Part print with two shaded views. Sizes in mm from the minimum x, y, z corner. A direction names the side the tool comes from. Round coordinates to 2 decimals unless told otherwise and drop trailing zeros. Order: outer loops, then holes, each group sorted by start corner. A loop starts at its lowest first (then second) coordinate and runs counter-clockwise, first axis right, second up. Notation, with made-up numbers: (41.5, 89) - (96.5, 89) arc R34 ccw to (96.5, 127) - close; hole circle Ø10 at (59, 81). An arc over 180 degrees is marked (long way). Use one line per item in the form item = value.
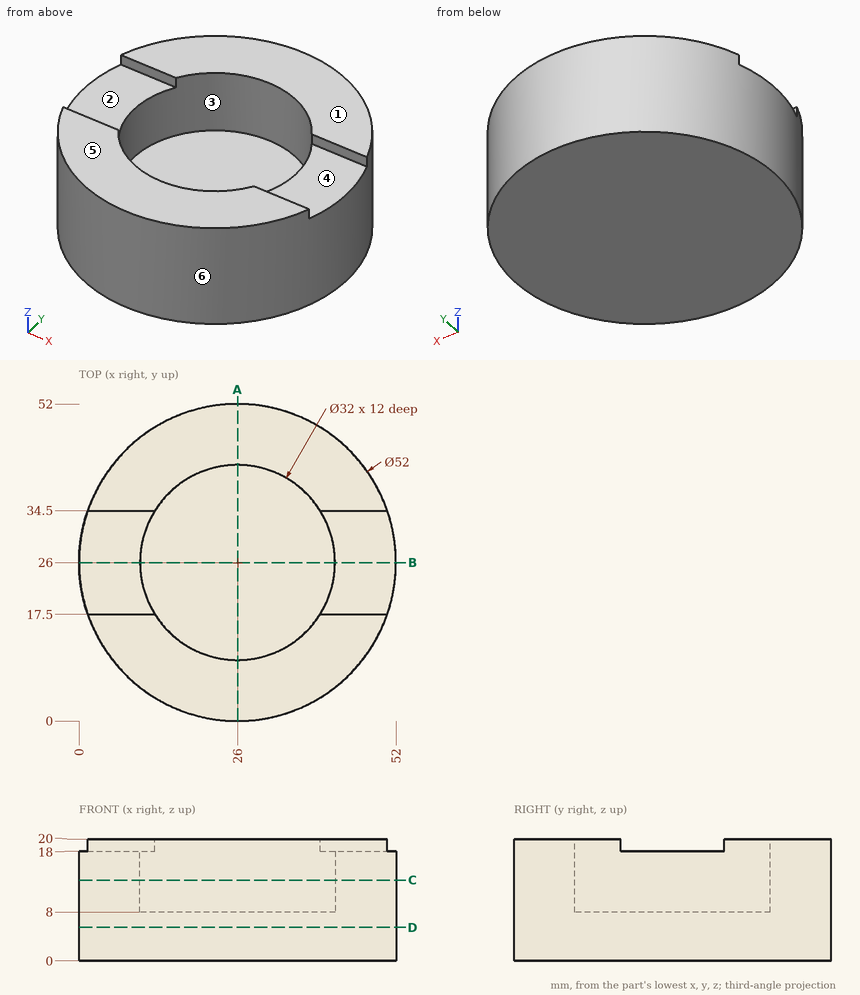
(1) Slice it at B-B on y = 26. Give the cut face in (x, z), then the cut area to 3 significant figures.
Report:
outline = (0, 0) - (52, 0) - (52, 18) - (42, 18) - (42, 8) - (10, 8) - (10, 18) - (0, 18) - close
area = 616 mm2
(2) Slice it at A-A on x = 26. Give the cut face in (y, z).
Report:
outline = (0, 0) - (52, 0) - (52, 20) - (42, 20) - (42, 8) - (10, 8) - (10, 20) - (0, 20) - close
(3) Pull direction Y, two halves, no side cores. Call the marked faces 3, 4, 5 and 6: released by +Y, released by -Y, zero draft, split by the parting line, or undercut.
Report:
face_3 = undercut
face_4 = undercut
face_5 = zero draft
face_6 = split by the parting line
(4) Probe probe 1 along Y at (x, z) = (26, 14.5); probe 2 along X at (y, z) = (20, 11.75); probe 3 along X at (y, z) = (18.5, 10.25). List the from-to ranges inside material, lowest first. Write a range as [from, to].
Report:
probe_1 = [0, 10], [42, 52]
probe_2 = [0.7, 11.17], [40.83, 51.3]
probe_3 = [1.11, 11.87], [40.13, 50.89]
(5) Slice it at D-D on z = 5.5. Give the cut face in (x, y), then the cut area to 3 significant figures.
Report:
outline = circle Ø52 at (26, 26)
area = 2,120 mm2
(6) Slice it at C-C on z = 13.25. Give the cut face in (x, y).
Report:
outline = circle Ø52 at (26, 26); hole circle Ø32 at (26, 26)
(7) Tool access for the marked faces 1 and 2: list every direction of +Z, -Z, +X, -X, +Y, -Y with a clear straight run to the whole face (end or side of a thin tool).
Report:
face_1 = +Z, +X, -X, +Y, -Y
face_2 = +Z, +X, -X
(8) Pin check, flat tips, straight feed: pin 1 (1 mm diameter, centred on x = 5.5, z = 19.5, fed in from -Y); pin 2 (9.5 mm diameter, centred on x = 26, y = 33, fed in from +Z); pin 3 (10 mm diameter, centred on x = 5.5, z = 15, fed in from -Y). Stop position of each tip, or through.
Report:
pin_1 = 9.39
pin_2 = 8
pin_3 = 5.13
